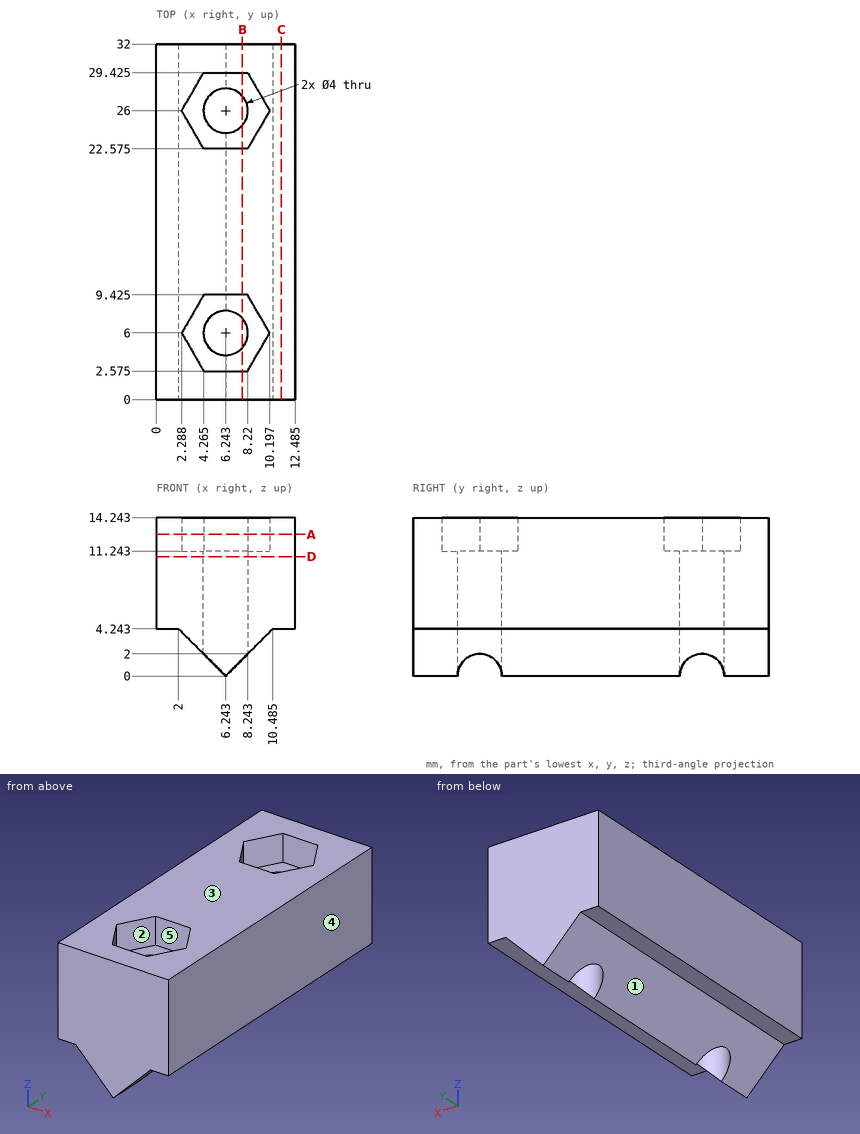
Source: three-view drawing plus pictorial views. Frame: mm from the lowest corner of the part. A direction names the side the tool comes from. Coordinates: 2 decimals unless noted, no trailing zeros. Write each loop counter-clockwise with the first axis right and the second up, starting at its lowest first coordinate (ties: lowest second). Pieces come first, ordered by that corner, then holes. Notation, with made-up numbers: (78.5, 48.25) - (125.5, 48.25) arc R20 ccw to (125.5, 74.25) - close; hole circle Ø11 at (-18, 85.5). An arc over 180 degrees is marked (long way). Return JSON: item names as keys, results as strings.
Item 1: Pull-direction query (X, two-part tool) for the marked faces 1, 2 and 3; classes: +X half, -X half, draft (parallel to the pull), parting line (faces both ways), or undercut.
Completed:
{"face 1": "-X half", "face 2": "undercut", "face 3": "draft"}
Item 2: Reachability of the marked faces 4 and 5 from +Z, -Z, +X, -X, +Y, -Y: full face, straight path, thin tool, end or side. Return the list, or none.
Completed:
{"face 4": "+Z, -Z, +X, +Y, -Y", "face 5": "+Z"}
Item 3: Section query C-C (x = 11.25). Output: boundary loops of the cut face in (y, z).
Completed:
{"outline": "(0, 4.24) - (32, 4.24) - (32, 14.24) - (0, 14.24) - close"}
Item 4: Line query: L1, parallel to Y at x = 5.5, z = 12.5 (1 decimal); L2, parallel to Y at x = 5.75, z = 4; L3, parallel to X at y = 6, z = 7.25 (1 decimal). Output: solid intervals per line, ascending.
Completed:
{"L1": "y = 0 to 2.6, 9.4 to 22.6, 29.4 to 32", "L2": "y = 0 to 4.06, 7.94 to 24.06, 27.94 to 32", "L3": "x = 0 to 4.2, 8.2 to 12.5"}
Item 5: Pin query (flat end, axial travel): pin 1 Ø1.6 at (x, y) = (1.5, 20.5) entering from -Z; pin 2 Ø3 at (x, z) = (10.5, 3.5) entering from +Y; pin 3 Ø2 at (x, y) = (12, 11.5) entering from -Z. Return the tip coordinate at first contact, or that it passes through.
Completed:
{"pin 1": "stops at z = 3.94", "pin 2": "stops at y = 32", "pin 3": "stops at z = 4.24"}
Item 6: Section query A-A (z = 12.75). Output: boundary loops of the cut face in (x, y) (1 decimal), and give its area (3 significant figures).
Completed:
{"outline": "(0, 0) - (12.5, 0) - (12.5, 32) - (0, 32) - close; hole (2.3, 6) - (4.3, 2.6) - (8.2, 2.6) - (10.2, 6) - (8.2, 9.4) - (4.3, 9.4) - close; hole (2.3, 26) - (4.3, 22.6) - (8.2, 22.6) - (10.2, 26) - (8.2, 29.4) - (4.3, 29.4) - close", "area": "318 mm2"}
Item 7: Section query D-D (z = 10.75). Output: boundary loops of the cut face in (x, y) (1 decimal).
Completed:
{"outline": "(0, 0) - (12.5, 0) - (12.5, 32) - (0, 32) - close; hole circle Ø4 at (6.2, 6); hole circle Ø4 at (6.2, 26)"}
Item 8: Section query B-B (x = 7.75). Output: boundary loops of the cut face in (y, z) (1 decimal), and give its area (3 significant figures).
Completed:
{"outline": "(0, 1.5) - (4.7, 1.5) - (4.7, 11.2) - (2.6, 11.2) - (2.6, 14.2) - (0, 14.2) - close; (7.3, 1.5) - (24.7, 1.5) - (24.7, 11.2) - (22.6, 11.2) - (22.6, 14.2) - (9.4, 14.2) - (9.4, 11.2) - (7.3, 11.2) - close; (27.3, 1.5) - (32, 1.5) - (32, 14.2) - (29.4, 14.2) - (29.4, 11.2) - (27.3, 11.2) - close", "area": "315 mm2"}
